from build123d import *

# Parameters (mm, degrees)
CROQUIS1_W               = 10
CROQUIS1_H               = 12
SALIENTE_EXTRUIR1_DEPTH  = 9
SALIENTE_EXTRUIR2_DEPTH  = 15
CROQUIS3_W               = 1
CROQUIS3_H               = 0.5
SALIENTE_EXTRUIR3_DEPTH  = 2
CROQUIS4_R               = 2.5000000000000004
SALIENTE_EXTRUIR4_DEPTH  = 2
CROQUIS5_R               = 1.95
SALIENTE_EXTRUIR5_DEPTH  = 0.6
SALIENTE_EXTRUIR9_DEPTH  = 10
CROQUIS7_W               = 15.000000000000002
CROQUIS7_H               = 7.000000000000002
CORTAR_EXTRUIR1_DEPTH    = 0.01
CROQUIS8_W               = 15.000000000000002
CROQUIS8_H               = 7.0000000000000036
CORTAR_EXTRUIR2_DEPTH    = 0.01
REDONDEO1_R              = 0.9
REDONDEO2_R              = 0.9
REDONDEO3_R              = 0.5
CROQUIS9_R               = 0.4628353533662974
SALIENTE_EXTRUIR7_DEPTH  = 0.01
REDONDEO4_R              = 0.09
REDONDEO6_R              = 1
SKETCH2_R                = 4.5
BOSS_EXTRUDE1_DEPTH      = 4
BOSS_EXTRUDE3_DEPTH      = 10
BOSS_EXTRUDE3_DEPTH_BACK = 1


with BuildPart() as part:
    # Croquis1 → Saliente-Extruir1 (new body)
    with BuildSketch(Plane.XY):
        with Locations((5, 6)):
            Rectangle(CROQUIS1_W, CROQUIS1_H)
    extrude(amount=SALIENTE_EXTRUIR1_DEPTH)

    # Croquis2 → Saliente-Extruir2 (add)
    with BuildSketch(Plane(origin=(0, 0, 0), x_dir=(-1, 0, 0), z_dir=(0, 0, -1))):
        with BuildLine():
            Line((-10, 9.5), (-10, 2.5))
            ThreePointArc((-10, 2.5), (-5, -0.10327780786685103), (0, 2.5000000000000004))
            Line((0, 2.5000000000000004), (0, 9.5))
            ThreePointArc((0, 9.5), (-5, 12.103277807866851), (-10, 9.5))
        make_face()
    extrude(amount=SALIENTE_EXTRUIR2_DEPTH)

    # Croquis3 → Saliente-Extruir3 (add)
    with BuildSketch(Plane(origin=(0, 0, -15), x_dir=(-1, 0, 0), z_dir=(0, 0, -1))):
        with Locations((-5.000000000000001, 9.748277807866852)):
            Rectangle(CROQUIS3_W, CROQUIS3_H)
        Polygon((-5.499999999999999, 1.520287769635288), (-4.499999999999999, 1.5202877696352886), (-4.499999999999999, 1.020287769635288), (-5.499999999999999, 1.020287769635288), align=None)
    extrude(amount=SALIENTE_EXTRUIR3_DEPTH)

    # Croquis4 → Saliente-Extruir4 (add)
    with BuildSketch(Plane(origin=(0, 0, -15), x_dir=(-1, 0, 0), z_dir=(0, 0, -1))):
        with Locations(Location((-5, 6, 0), (0, 0, 180))):
            Circle(CROQUIS4_R)
    extrude(amount=SALIENTE_EXTRUIR4_DEPTH)

    # Croquis5 → Saliente-Extruir5 (add)
    with BuildSketch(Plane.XY.offset(9)):
        with Locations(Location((5, 6, 0), (0, 0, 180))):
            Circle(CROQUIS5_R)
    extrude(amount=SALIENTE_EXTRUIR5_DEPTH)

    # Croquis6 → Saliente-Extruir9 (add)
    with BuildSketch(Plane.XY.offset(9.6)):
        with BuildLine():
            Line((3.8819660112501033, 6.999999999999999), (6.118033988749897, 6.999999999999999))
            ThreePointArc((6.118033988749897, 6.999999999999999), (5, 4.499999999999999), (3.8819660112501033, 6.999999999999999))
        make_face()
    extrude(amount=SALIENTE_EXTRUIR9_DEPTH)

    # Croquis7 → Cortar-Extruir1 (cut)
    with BuildSketch(Plane(origin=(10, 0, 0), x_dir=(0, 0, -1), z_dir=(1, 0, 0))):
        with Locations((7.500000000000001, 5.999999999999999)):
            Rectangle(CROQUIS7_W, CROQUIS7_H)
    extrude(amount=-CORTAR_EXTRUIR1_DEPTH, mode=Mode.SUBTRACT)

    # Croquis8 → Cortar-Extruir2 (cut)
    with BuildSketch(Plane.ZY):
        with Locations((-7.500000000000001, 5.999999999999998)):
            Rectangle(CROQUIS8_W, CROQUIS8_H)
    extrude(amount=-CORTAR_EXTRUIR2_DEPTH, mode=Mode.SUBTRACT)

    # Redondeo1
    redondeo1_edges = [part.edges().sort_by_distance(p)[0] for p in [
        (9.99, 6, -15),
        (0.01, 5.999999999999998, -15),
    ]]
    fillet(redondeo1_edges, radius=REDONDEO1_R)

    # Redondeo2
    # the kernel refuses this fillet: 0.9 mm, written as the material it takes off along each edge
    with BuildSketch(Plane(origin=(5, 6.000000000000001, -15), x_dir=(-0.9708964954680348, 0.23949946782381015, 0), z_dir=(-0.23949946782381015, -0.9708964954680348, 0))) as redondeo2_piece_1:
        with BuildLine():
            CenterArc((6.103277807866849 - REDONDEO2_R, -REDONDEO2_R), REDONDEO2_R, 0, 90)
            Line((6.103277807866849, -REDONDEO2_R), (6.103277807866849, 0))
            Line((6.103277807866849, 0), (6.103277807866849 - REDONDEO2_R, 0))
        make_face()
    revolve(axis=Axis((5, 6.000000000000001, -15), (0, 0, -1)), revolution_arc=152.28599911771772, mode=Mode.SUBTRACT)
    with BuildSketch(Plane(origin=(5, 6, -15), x_dir=(0.9708964954680347, -0.23949946782381032, 0), z_dir=(0.23949946782381032, 0.9708964954680347, 0))) as redondeo2_piece_2:
        with BuildLine():
            CenterArc((6.103277807866849 - REDONDEO2_R, -REDONDEO2_R), REDONDEO2_R, 0, 90)
            Line((6.103277807866849 - REDONDEO2_R, 0), (6.103277807866849, 0))
            Line((6.103277807866849, 0), (6.103277807866849, -REDONDEO2_R))
        make_face()
    revolve(axis=Axis((5, 6, -15), (0, 0, -1)), revolution_arc=152.2859991177177, mode=Mode.SUBTRACT)

    # Redondeo3
    redondeo3_edges = [part.edges().sort_by_distance(p)[0] for p in [
        (2.4999999999999996, 5.999999999999999, -17),
    ]]
    fillet(redondeo3_edges, radius=REDONDEO3_R)

    # Croquis9 → Saliente-Extruir7 (add)
    with BuildSketch(Plane(origin=(0, 0, -17), x_dir=(-1, 0, 0), z_dir=(0, 0, -1))):
        with Locations((-5, 6)):
            Circle(CROQUIS9_R)
    extrude(amount=SALIENTE_EXTRUIR7_DEPTH)

    # Redondeo4
    redondeo4_edges = [part.edges().sort_by_distance(p)[0] for p in [
        (5.500000000000001, 9.998277807866852, -16),
        (5.500000000000001, 9.498277807866852, -16),
        (4.500000000000001, 9.498277807866852, -16),
        (4.500000000000001, 9.998277807866852, -16),
        (5.500000000000001, 9.748277807866852, -17),
        (5.000000000000001, 9.498277807866852, -17),
        (4.500000000000001, 9.748277807866852, -17),
        (5.000000000000001, 9.998277807866852, -17),
        (5.499999999999999, 1.520287769635288, -16),
        (5.499999999999999, 1.020287769635288, -16),
        (4.499999999999999, 1.020287769635288, -16),
        (4.499999999999999, 1.5202877696352886, -16),
        (5.499999999999999, 1.270287769635288, -17),
        (4.999999999999999, 1.020287769635288, -17),
        (4.499999999999999, 1.2702877696352883, -17),
        (4.999999999999999, 1.5202877696352883, -17),
    ]]
    fillet(redondeo4_edges, radius=REDONDEO4_R)

    # Redondeo6
    redondeo6_edges = [part.edges().sort_by_distance(p)[0] for p in [
        (10, 12, 4.5),
        (10, 0, 4.5),
        (0, 0, 4.5),
        (0, 12, 4.5),
    ]]
    fillet(redondeo6_edges, radius=REDONDEO6_R)

    # Sketch2 → Boss-Extrude1 (add)
    with BuildSketch(Plane(origin=(0, 0, -17), x_dir=(-1, 0, 0), z_dir=(0, 0, -1))):
        with Locations((-5, 6)):
            Circle(SKETCH2_R)
    extrude(amount=BOSS_EXTRUDE1_DEPTH)

    # Sketch3 → Boss-Extrude3 (add, two sides: drawn at the far end of the back side and taken through both)
    with BuildSketch(Plane.ZY.offset(-0.01).offset(-BOSS_EXTRUDE3_DEPTH_BACK)):
        Polygon((-14.100000000000003, 12.103277807866851), (-21.100000000000005, 12.103277807866851), (-21.1, 0), (-14.100000000000003, 0), align=None)
    extrude(amount=BOSS_EXTRUDE3_DEPTH + BOSS_EXTRUDE3_DEPTH_BACK)


solid = part.part
Could you check a few things on this model? Use its own coordinates, in mm. A direction names the side the tool comes from. Give positions to 0.01 mm unless a question says otherwise; leave off trailing zeros. Loops run counter-clockwise (first coordinate to the right, second up) from the corner with the lowest first, then second, coordinate; pieces in that order, holes last. Notation, with made-up numbers: (-16.75, 46.25) -> (42.25, 46.25) arc R12 ccw to (42.25, 58.25) -> close; hole circle Ø3 at (58, 36). An arc over 180 degrees is marked (long way). Return JSON: item names as keys, results as strings.
Item 1: Which directions (+Z, -Z, +X, -X, +Y, -Y) give clear straight access to the entire face, cutting with the end or side of a thin tool? Please do faces 1 (the flat face through (1, 11, 0)), 2 (the flat face through (7.2, 7.1, -17)), 3 (the flat face through (5, 6, -21)), 4 (the flat face through (5, 9.498, -16)), 5 (the flat face through (5, 9.998, -16)).
Geometry results:
{"face 1": "-X, +Y", "face 2": "none", "face 3": "-Z, +X, +Y, -Y", "face 4": "+X", "face 5": "+X, +Y"}
Item 2: I'm going to push flat-ended pins straight in: pin 1 (1 mm diameter, centred on x = 7.5, y = 7.5, fed in from -Z); pin 2 (3.5 mm diameter, centred on y = 5, z = -5, fed in from -X); pin 3 (5.5 mm diameter, centred on x = -7, z = -17, fed in from -Y). Where does each tip first touch, or does it pass through?
Geometry results:
{"pin 1": "stops at z = -21", "pin 2": "stops at x = 0.01", "pin 3": "stops at y = 0"}
Item 3: If we section it at B-B on x = -7.5: List the corners of the cut face in (y, z) for me.
Geometry results:
{"outline": "(0, -21.1) -> (12.1, -21.1) -> (12.1, -14.1) -> (0, -14.1) -> close"}
Item 4: I need wall thicknesses on L1, parallel to Z at x = 5.75, y = 9.5; L2, parallel to Y at x = 7, z = 5; L3, parallel to X at y = 5.5, z = -4. Which ranges of each line are inside material? Lowest first, please. Write a range as from..to.
Geometry results:
{"L1": "z = -21..-17, -15..9", "L2": "y = 0..12", "L3": "x = 0.01..9.99"}
Item 5: We'd pull the mould along Z, two halves only. Please class faces 6 (the flat face through (1, 1, 0)), 7 (the flat face through (5, 6, 19.6)), 8 (the flat face through (-9.99, 6, -18)): +Z half, -Z half, draft (parallel to the pull), parting line (faces both ways), or undercut.
Geometry results:
{"face 6": "undercut", "face 7": "+Z half", "face 8": "draft"}
